Model file for the job. Use its own axes, mm. A direction names the side the tool comes from. Round coordinates to 2 decimals unless told otherwise and drop trailing zeros. Write item = value, one per line.
```python
from build123d import *

# Parameters (mm, degrees)
F0_W     = 98.3085063696
F0_H     = 59.0165173113
F0_W_2   = 92.3085063696
F0_H_2   = 53.0165173113
F1_DEPTH = 8
F2_DEPTH = 15
F3_R     = 4.3592981544
F3_R_2   = 1.7500302992
F4_DEPTH = 8.001
F3_R_3   = 5
F3_R_4   = 4
F5_DEPTH = 6
F6_R     = 2.54
F7_R     = 1.7500302992
F8_DEPTH = 3
F9_R     = 3
F10_R    = 2.99999


# Not quite as in the source:
# - a fillet or chamfer that OpenCascade refuses, or shapes differently, is made with other operations: its cross-section is extruded or revolved along the edge and cut away or added
# - a fillet or chamfer is up to 0.001 mm smaller than in the source, because OpenCascade refuses the exact size


with BuildPart() as f1:
    # F0 (on Front) → F1 (new body)
    with BuildSketch(Plane.XZ):
        Rectangle(F0_W, F0_H)
        Rectangle(F0_W_2, F0_H_2, mode=Mode.SUBTRACT)
        Rectangle(F0_W_2, F0_H_2)
    extrude(amount=F1_DEPTH)

    # F0 (on Front) → F2 (join)
    with BuildSketch(Plane.XZ):
        Rectangle(F0_W, F0_H)
        Rectangle(F0_W_2, F0_H_2, mode=Mode.SUBTRACT)
    extrude(amount=F2_DEPTH)

    # F3 (on face) → F4 (cut, through all)
    with BuildSketch(Plane.XZ.offset(8)):
        Circle(F3_R)
        with Locations((5.6447647512, 5.1466971636)):
            Circle(F3_R_2)
        with Locations((-5.6447647512, 5.1466971636)):
            Circle(F3_R_2)
        with Locations((-5.6447647512, -5.1466971636)):
            Circle(F3_R_2)
        with Locations((5.6447647512, -5.1466971636)):
            Circle(F3_R_2)
    extrude(amount=-F4_DEPTH, mode=Mode.SUBTRACT)

    # F3 (on face) → F5 (join)
    with BuildSketch(Plane.XZ.offset(8)):
        with Locations((-24.5116613805, 0)):
            Circle(F3_R_3)
        with Locations((-24.5116613805, 0)):
            Circle(F3_R_4, mode=Mode.SUBTRACT)
        with Locations((24.5116613805, 0)):
            Circle(F3_R_3)
        with Locations((24.5116613805, 0)):
            Circle(F3_R_4, mode=Mode.SUBTRACT)
    extrude(amount=F5_DEPTH)

    # F6
    f6_edges = [f1.edges().sort_by_distance(p)[0] for p in [
        (-29.511661, -8, 0),
        (19.511661, -8, 0),
        (0, -8, -26.508259),
        (46.154253, -8, 0),
        (-46.154253, -8, 0),
        (0, -8, 26.508259),
    ]]
    fillet(f6_edges, radius=F6_R)

    # F7 (on face) → F8 (cut)
    with BuildSketch(Plane.XZ.offset(8)):
        Polygon((-2.9085768434, 5.0357150996), (-4.2244093493, 7.4292570353), (-6.9551937235, 7.4864836259), (-8.3701455918, 5.1501682809), (-7.054313086, 2.7566263452), (-4.3235287118, 2.6993997546), align=None)
        with Locations((-5.6447647512, 5.1466971636)):
            Circle(F7_R, mode=Mode.SUBTRACT)
        Polygon((8.3701455918, 5.1501682809), (6.9551937235, 7.4864836259), (4.2244093493, 7.4292570353), (2.9085768434, 5.0357150996), (4.3235287118, 2.6993997546), (7.054313086, 2.7566263452), align=None)
        with Locations((5.6447647512, 5.1466971636)):
            Circle(F7_R, mode=Mode.SUBTRACT)
        Polygon((4.3235287118, -2.6993997546), (2.9085768434, -5.0357150996), (4.2244093493, -7.4292570353), (6.9551937235, -7.4864836259), (8.3701455918, -5.1501682809), (7.054313086, -2.7566263452), align=None)
        with Locations((5.6447647512, -5.1466971636)):
            Circle(F7_R, mode=Mode.SUBTRACT)
        Polygon((-2.9085768434, -5.0357150996), (-4.3235287118, -2.6993997546), (-7.054313086, -2.7566263452), (-8.3701455918, -5.1501682809), (-6.9551937235, -7.4864836259), (-4.2244093493, -7.4292570353), align=None)
        with Locations((-5.6447647512, -5.1466971636)):
            Circle(F7_R, mode=Mode.SUBTRACT)
    extrude(amount=-F8_DEPTH, mode=Mode.SUBTRACT)

    # F9
    f9_edges = [f1.edges().sort_by_distance(p)[0] for p in [
        (0, 0, 29.508259),
        (49.154253, 0, 0),
        (0, 0, -29.508259),
        (-49.154253, 0, 0),
    ]]
    fillet(f9_edges, radius=F9_R)

    # F10 (radius 3 in the source; OpenCascade refuses exactly that, so slightly less here)
    f10_edges = [f1.edges().sort_by_distance(p)[0] for p in [
        (0, -15, -29.508259),
        (49.154253, -15, 0),
        (-49.154253, -15, 0),
        (0, -15, 29.508259),
    ]]
    fillet(f10_edges, radius=F10_R)

    # F11: fillet of radius 2 on 2 edges, made by hand

    # F11_s1 → F11_t2 (revolve, cut)
    with BuildSketch(Plane.XY):
        with BuildLine():
            ThreePointArc((29.5120613805, -12.2673917434), (29.2440686279, -13.2678330874), (28.5118614771, -14.0003463544))
            Line((28.5118614771, -14.0003463544), (28.6119780552, -14.1736418155))
            ThreePointArc((28.6119780552, -14.1736418155), (29.0117614288, -14.2001365685), (29.5116613805, -14.2001365685))
            Line((29.5116613805, -14.2001365685), (29.7117979491, -14))
            ThreePointArc((29.7117979491, -14), (29.7117979491, -13.1336958717), (29.7121979491, -12.2673917434))
            Line((29.7121979491, -12.2673917434), (29.5120613805, -12.2673917434))
        make_face()
    revolve(axis=Axis((24.5116613805, -14, 0), (0, -1, 0)), mode=Mode.SUBTRACT)

    # F11_s3 → F11_t4 (revolve, cut)
    with BuildSketch(Plane.XY):
        with BuildLine():
            ThreePointArc((-19.5112613805, -12.2673917434), (-19.7792541332, -13.2678330874), (-20.511461284, -14.0003463544))
            Line((-20.511461284, -14.0003463544), (-20.4113447058, -14.1736418155))
            ThreePointArc((-20.4113447058, -14.1736418155), (-20.0115613323, -14.2001365685), (-19.5116613805, -14.2001365685))
            Line((-19.5116613805, -14.2001365685), (-19.311524812, -14))
            ThreePointArc((-19.311524812, -14), (-19.311524812, -13.1336958717), (-19.311124812, -12.2673917434))
            Line((-19.311124812, -12.2673917434), (-19.5112613805, -12.2673917434))
        make_face()
    revolve(axis=Axis((-24.5116613805, -14, 0), (0, -1, 0)), mode=Mode.SUBTRACT)


solid = f1.part
```
1) 3-axis set-ups, long thin cutter, end or side, ignore diameter. For faces 1 (the face through (49.154, -7, 0)), 2 (the face through (29.28, -11.41, 1.5)): which of +Z, -Z, +X, -X, +Y, -Y reach the whole face in a straight line?
Conclusion:
face_1 = +Z, -Z, +X, +Y, -Y
face_2 = -Y
2) Wall check: line 1 along Z through (x, y) = (-6, -11.75); line 2 along X through (y, z) = (-12, 18.5); line 3 along Z through (x, y) = (21, -8.5). Give the ranges that are in metal, low to high.
Conclusion:
line_1 = -29.51 to -26.51, 26.51 to 29.51
line_2 = -49.15 to -46.15, 46.15 to 49.15
line_3 = -29.51 to -25.48, -4.9 to -1.92, 1.92 to 4.9, 25.48 to 29.51
3) Mould opens along Z. For faces 3 (the face through (0.69, -14.14, 28.61)), 4 (the face through (-1, 0, 6)), 5 (the face through (5, -5, 3)) say: +Z half, -Z half, draft (parallel to the pull), parting line (faces both ways), or undercut.
Conclusion:
face_3 = +Z half
face_4 = draft
face_5 = undercut
4) Flat gauge pins, fed straight in: pin 1 Ø4 at (x, z) = (-6.5, 6) entering from -Y; pin 2 Ø9 at (x, z) = (26, 0.5) entering from -Y; pin 3 Ø2 at (x, z) = (-5.64, 5.15) entering from -Y; pin 4 Ø1 at (y, z) = (-13.5, -3.5) entering from -X. Where does each tip first touch, or does it go through?
Conclusion:
pin_1 = -8
pin_2 = -14
pin_3 = through
pin_4 = -48.98
